from build123d import *

# Parameters (mm, degrees)
F0_W      = 800
F0_H      = 400
F1_DEPTH  = 50
F2_R      = 90
F3_DEPTH  = 300
F4_R      = 20
F5_DEPTH  = 200
F6_R      = 60
F7_DEPTH  = 25
F9_DEPTH  = 20
F10_R     = 30
F11_DEPTH = 40
F12_W     = 120
F12_H     = 60
F13_DEPTH = 775
F14_R     = 40
F15_DEPTH = 150
F16_W     = 500
F16_H     = 500
F17_DEPTH = 50
F18_R     = 10
F19_DEPTH = 130
F25_W     = 60
F25_H     = 60
F26_DEPTH = 600


with BuildPart() as f1:
    # F0 (on Front) → F1 (new body, symmetric)
    with BuildSketch(Plane.XZ):
        Rectangle(F0_W, F0_H)
    extrude(amount=F1_DEPTH, both=True)

    # F2 (on face) → F3 (join)
    with BuildSketch(Plane.XZ.offset(50)):
        Circle(F2_R)
    extrude(amount=F3_DEPTH)

    # F4 (on Top) → F5 (join)
    with BuildSketch(Plane.XY):
        with Locations((0, -280)):
            Circle(F4_R)
    extrude(amount=F5_DEPTH)

    # F6 (on Right) → F7 (join, symmetric)
    with BuildSketch(Plane.YZ):
        with Locations((-280, 245)):
            Circle(F6_R)
    extrude(amount=F7_DEPTH, both=True)

    # F8 (on face) → F9 (join)
    with BuildSketch(Plane.XZ.offset(50)):
        Polygon((-318.2610926981, -31.6291403548), (-281.7389073019, -31.6291403548), (-263.4778146039, 0), (-281.7389073019, 31.6291403548), (-318.2610926981, 31.6291403548), (-336.5221853961, 0), align=None)
        Polygon((281.7389073019, 31.6291403548), (263.4778146039, 0), (281.7389073019, -31.6291403548), (318.2610926981, -31.6291403548), (336.5221853961, 0), (318.2610926981, 31.6291403548), align=None)
    extrude(amount=F9_DEPTH)

    # F10 (on face) → F11 (cut)
    with BuildSketch(Plane(origin=(0, 50, 0), x_dir=(-1, 0, 0), z_dir=(0, 1, 0))):
        with Locations((-300, 0)):
            Circle(F10_R)
        with Locations((300, 0)):
            Circle(F10_R)
    extrude(amount=-F11_DEPTH, mode=Mode.SUBTRACT)

    # F12 (on face) → F13 (join)
    with BuildSketch(Plane(origin=(0, 0, -200), x_dir=(1, 0, 0), z_dir=(0, 0, -1))):
        with Locations((335, -15)):
            Rectangle(F12_W, F12_H)
        with Locations((-335, -15)):
            Rectangle(F12_W, F12_H)
    extrude(amount=F13_DEPTH)

    # F14 (on face) → F15 (join)
    with BuildSketch(Plane(origin=(0, 50, 0), x_dir=(-1, 0, 0), z_dir=(0, 1, 0))):
        Circle(F14_R)
    extrude(amount=F15_DEPTH)

    # F16 (on face) → F17 (join)
    with BuildSketch(Plane(origin=(0, 200, 0), x_dir=(-1, 0, 0), z_dir=(0, 1, 0))):
        Rectangle(F16_W, F16_H)
    extrude(amount=F17_DEPTH)

    # F18 (on face) → F19 (join)
    with BuildSketch(Plane(origin=(-250, 0, 0), x_dir=(0, -1, 0), z_dir=(-1, 0, 0))):
        with Locations((-225, 50)):
            Circle(F18_R)
    extrude(amount=F19_DEPTH)

    # F22 (on offset) → F23 (revolve)
    with BuildSketch(Plane(origin=(0, 225, 0), x_dir=(-1, 0, 0), z_dir=(0, 1, 0))):
        with BuildLine():
            Line((340, 40), (260, 40))
            Line((260, 40), (260, 20))
            add(Edge.make_bspline(
                [(260, 20), (273.2887466803, 26.2524876464), (300.1899032178, 35.4131948165), (326.622332785, 26.2265646487), (340, 20)],
                knots=[0, 0, 0, 0, 0.5006142666, 1, 1, 1, 1], degree=3))
            Line((340, 20), (340, 40))
        make_face()
    revolve(axis=Axis((-250, 225, 50), (1, 0, 0)))

    # F24: F1 across plane


with BuildPart() as f1_1:
    add(f1.part)
    add(f1.part.mirror(Plane.YZ))

    # F25 (on face) → F26 (join)
    with BuildSketch(Plane(origin=(275, 0, 0), x_dir=(0, -1, 0), z_dir=(-1, 0, 0))):
        with Locations((-15, -550)):
            Rectangle(F25_W, F25_H)
    extrude(amount=F26_DEPTH)


solid = f1_1.part
Check sheet for the modelled part. Datum: model origin and axes. Units: mm. A direction names the side the tool comes from. Round coordinates to 2 decimals unless told otherwise and drop trailing zeros. Order: outer loops, then holes, each group sorted by start corner. A loop starts at its lowest first (then second) coordinate and runs counter-clockwise, first axis right, second up.
Q1. Cross-section at C-C, the plane x = 0. Enter the section's corners in (y, z), plus the area to 3 significant figures.
Filled sheet:
outline: (-350, -90) - (-50, -90) - (-50, -200) - (50, -200) - (50, -40) - (200, -40) - (200, -250) - (250, -250) - (250, 250) - (200, 250) - (200, 40) - (50, 40) - (50, 200) - (-50, 200) - (-50, 90) - (-260, 90) - (-260, 188.43) arc R60 ccw (long way) to (-300, 188.43) - (-300, 90) - (-350, 90) - close; (-15, -580) - (45, -580) - (45, -520) - (-15, -520) - close
area: 150,000 mm2
Q2. Scan lines: L1, parallel to X at y = 29, z = 0; L2, parallel to Z at x = 172, y = 23; L3, parallel to Y at x = -168.5, z = -166.5. Record each from-to range of solid material in increasing order.
Filled sheet:
L1: x = -400 to -330, -270 to 270, 330 to 400
L2: z = -580 to -520, -200 to 200
L3: y = -50 to 50, 200 to 250
Q3. Set-up check for faces 4 (the face through (-275, 15, -358)), 5 (the face through (8.67, 123.95, -39.05)), 6 (the face through (395, 15, -582)), 7 (the face through (300, 10, 0)), 8 (the face through (4, 15, -580)): record each of +Z, -Z, +X, -X, +Y, -Y from which the full face is reachable in a straight line by a thin tool's end or side.
Filled sheet:
face 4: +Y, -Y
face 5: none
face 6: -Z, +X, +Y, -Y
face 7: +Y
face 8: -Z, +Y, -Y
Q4. Cross-section at D-D, the plane y = -280. Enter the section's corners in (x, z), plus the area to 3 significant figures.
Filled sheet:
outline: (-25, 185) - (-20, 185) - (-20, 87.75) arc R90 ccw (long way) to (20, 87.75) - (20, 185) - (25, 185) - (25, 305) - (-25, 305) - close
area: 35,300 mm2
Q5. Cross-section at B-B, the plane z = -770.5. Enter the section's corners in (x, y).
Filled sheet:
outline: (-395, -15) - (-275, -15) - (-275, 45) - (-395, 45) - close; (275, -15) - (395, -15) - (395, 45) - (275, 45) - close
Q6. Draft check along Z on faces 1 (the face through (334, 15, -975)), 2 (the face through (275, 15, -358)), 3 (the face through (-340, 225, 37)). Enter one of: pulls with the +Z half, pulls with the -Z half, needs draft (parallel to the pull), parting line crosses it, or undercut.
Filled sheet:
face 1: pulls with the -Z half
face 2: undercut
face 3: needs draft
Q7. Cross-section at A-A, the plane z = 145. Enter the section's corners in (x, y).
Filled sheet:
outline: (-400, -50) - (400, -50) - (400, 50) - (-400, 50) - close; (-250, 200) - (250, 200) - (250, 250) - (-250, 250) - close; circle Ø40 at (0, -280)
Q8. Depth check by flat-ended pin: P1, Ø16, axis at x = -306.5, y = -56.5, coming from the -Z side; P2, Ø18, axis at y = 15, z = -725, coming from the +X side; P3, Ø4, axis at x = 135.5, y = 45.5, coming from the -Z side. Enter the tip coordinate at first touch or a pass-through.
Filled sheet:
P1: stops at z = -200
P2: stops at x = 395
P3: stops at z = -580
